Work out the finished part from the listing and answer in its coordinate system (mm). Face numbers are marked on the shaded views. A direction names the side the tool comes from. Give positions to 0.01 mm unless a question says otherwise; leave off trailing zeros. Loops run counter-clockwise (first coordinate to the right, second up) from the corner with the lowest first, then second, coordinate; pieces in that order, holes last. Notation, with made-up numbers: M 1,43.5 L 41,43.5 A16 cw 41,55.5 Z; hole C 44,54.25 d2. An arc over 180 degrees is marked long. Answer in a Markdown table with one row per item. Add a question column.
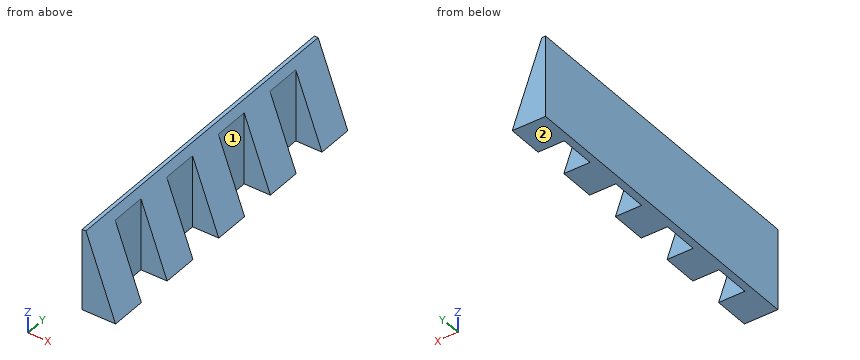
from build123d import *

# Parameters (mm, degrees)
PAD018_DEPTH    = 158.75
SKETCH026_W     = 12.88
SKETCH026_H     = 17.638889
POCKET007_DEPTH = 45
SKETCH027_W     = 5
SKETCH027_H     = 5
POCKET008_DEPTH = 200


with BuildPart() as part:
    # Sketch025 → Pad018 (new body)
    with BuildSketch(Plane.XZ):
        Polygon((0, 0), (0, 45), (16.38, 0), align=None)
    extrude(amount=PAD018_DEPTH)

    # Sketch026 (on Face3 of Pad018) → Pocket007 (cut)
    with BuildSketch(Plane(origin=(0, 0, 0), x_dir=(1, 0, 0), z_dir=(0, 0, -1))):
        with Locations((9.94, 26.458333)):
            Rectangle(SKETCH026_W, SKETCH026_H)
        with Locations((9.94, 132.291666)):
            Rectangle(SKETCH026_W, SKETCH026_H)
        with Locations((9.94, 97.013888)):
            Rectangle(SKETCH026_W, SKETCH026_H)
        with Locations((9.94, 61.736111)):
            Rectangle(SKETCH026_W, SKETCH026_H)
    extrude(amount=-POCKET007_DEPTH, mode=Mode.SUBTRACT)

    # Sketch027 (on Face5 of Pocket007) → Pocket008 (cut)
    with BuildSketch(Plane.XZ.offset(158.75)):
        with Locations((2.5, 42.5)):
            Rectangle(SKETCH027_W, SKETCH027_H)
    extrude(amount=-POCKET008_DEPTH, mode=Mode.SUBTRACT)


solid = part.part
(1) Section B-B, the plane z = 20 is taken. Determine the outline of the cut face in (x, y).
(2) Section C-C, the plane y = -66.5 is taken. Determine the outline of the cut face in (x, z).
(3) Each of these flat-tipped pins is pushed along its axis until it touches: P1, Ø9, axis at y = -62.5, z = 10, coming from the +X side; P2, Ø2, axis at x = 5.5, z = 34, coming from the -Y side; P3, Ø14, axis at y = -92.5, z = 17.5, coming from the +X side. Where does it stop, or does it pass through?
(4) Which of the six approach directions +Z, -Z, +X, -X, +Y, -Y give full straight-line access (tool end or side, diameter ignored) to the marked faces 1 and 2?
(5) Section A-A, the plane x = 7.5 is taken. Determine the outline of the cut face in (y, z).
(6) Section D-D, the plane z = 5 is taken. Determine the outline of the cut face in (x, y), and give its area (3 significant figures).
(7) Consider line 1 along Y through (x, z) = (9, 16); line 2 along X through (y, z) = (-95, 6); line 3 along X through (y, z) = (-15, 36.5). Determine where each line is inside the solid, lowest interval first. Write a range as from..to.
Numbers:
| question | item | result |
|---|---|---|
| 1 | outline | M 0,-158.75 L 9.1,-158.75 L 9.1,-141.11 L 3.5,-141.11 L 3.5,-123.47 L 9.1,-123.47 L 9.1,-105.83 L 3.5,-105.83 L 3.5,-88.19 L 9.1,-88.19 L 9.1,-70.56 L 3.5,-70.56 L 3.5,-52.92 L 9.1,-52.92 L 9.1,-35.28 L 3.5,-35.28 L 3.5,-17.64 L 9.1,-17.64 L 9.1,0 L 0,0 Z |
| 2 | outline | M 0,0 L 3.5,0 L 3.5,35.38 L 1.82,40 L 0,40 Z |
| 3 | P1 | stops at x = 3.5 |
| 3 | P2 | passes through |
| 3 | P3 | stops at x = 12.02 |
| 4 | face 1 | +Z, -Z, +X |
| 4 | face 2 | -Z, +X, -X, +Y, -Y |
| 5 | outline | M -158.75,0 L -141.11,0 L -141.11,24.4 L -158.75,24.4 Z; M -123.47,0 L -105.83,0 L -105.83,24.4 L -123.47,24.4 Z; M -88.19,0 L -70.56,0 L -70.56,24.4 L -88.19,24.4 Z; M -52.92,0 L -35.28,0 L -35.28,24.4 L -52.92,24.4 Z; M -17.64,0 L 0,0 L 0,24.4 L -17.64,24.4 Z |
| 6 | outline | M 0,-158.75 L 14.56,-158.75 L 14.56,-141.11 L 3.5,-141.11 L 3.5,-123.47 L 14.56,-123.47 L 14.56,-105.83 L 3.5,-105.83 L 3.5,-88.19 L 14.56,-88.19 L 14.56,-70.56 L 3.5,-70.56 L 3.5,-52.92 L 14.56,-52.92 L 14.56,-35.28 L 3.5,-35.28 L 3.5,-17.64 L 14.56,-17.64 L 14.56,0 L 0,0 Z |
| 6 | area | 1,530 mm² |
| 7 | line 1 | y = -158.75..-141.11, -123.47..-105.83, -88.19..-70.56, -52.92..-35.28, -17.64..0 |
| 7 | line 2 | x = 0..3.5 |
| 7 | line 3 | x = 0..3.09 |
